from build123d import *

# Parameters (mm, degrees)
ESQUISSE1_W             = 4
ESQUISSE1_H             = 2
BASE_EXTRUSION_DEPTH    = 2
BOSS_EXTRU_1_DEPTH      = 0.5
BOSS_EXTRU_2_DEPTH      = 0.5
ESQUISSE4_W             = 5.5
ESQUISSE4_H             = 3.5
ESQUISSE5_W             = 4
ESQUISSE5_H             = 2
CONG_1_R                = 0.5
ESQUISSE6_W             = 2.5
ESQUISSE6_H             = 1
ENL_V_MAT_EXTRU_1_DEPTH = 8.5


with BuildPart() as part:
    # Esquisse1 → Base-Extrusion (new body)
    with BuildSketch(Plane.XY):
        Rectangle(ESQUISSE1_W, ESQUISSE1_H)
    extrude(amount=BASE_EXTRUSION_DEPTH)

    # Esquisse2 → Boss.-Extru.1 (add)
    with BuildSketch(Plane(origin=(0, 0, 0), x_dir=(-1, 0, 0), z_dir=(0, 0, -1))):
        with BuildLine():
            Line((-3, 2.5), (3, 2.5))
            ThreePointArc((3, 2.5), (3.353553391, 2.353553391), (3.5, 2))
            Line((3.5, 2), (3.5, -2))
            ThreePointArc((3.5, -2), (3.353553391, -2.353553391), (3, -2.5))
            Line((3, -2.5), (-3, -2.5))
            ThreePointArc((-3, -2.5), (-3.353553391, -2.353553391), (-3.5, -2))
            Line((-3.5, -2), (-3.5, 2))
            ThreePointArc((-3.5, 2), (-3.353553391, 2.353553391), (-3, 2.5))
        make_face()
    extrude(amount=BOSS_EXTRU_1_DEPTH)

    # Esquisse3 → Boss.-Extru.2 (add)
    with BuildSketch(Plane.XY.offset(2)):
        with BuildLine():
            Line((-3, -2.5), (3, -2.5))
            ThreePointArc((3, -2.5), (3.353553391, -2.353553391), (3.5, -2))
            Line((3.5, -2), (3.5, 2))
            ThreePointArc((3.5, 2), (3.353553391, 2.353553391), (3, 2.5))
            Line((3, 2.5), (-3, 2.5))
            ThreePointArc((-3, 2.5), (-3.353553391, 2.353553391), (-3.5, 2))
            Line((-3.5, 2), (-3.5, -2))
            ThreePointArc((-3.5, -2), (-3.353553391, -2.353553391), (-3, -2.5))
        make_face()
    extrude(amount=BOSS_EXTRU_2_DEPTH)

    # Esquisse4 → Boss.-Lissage1 section 0
    with BuildSketch(Plane.XY.offset(2.5)):
        Rectangle(ESQUISSE4_W, ESQUISSE4_H)
    # Esquisse5 → Boss.-Lissage1 section 1
    with BuildSketch(Plane.XY.offset(7)):
        Rectangle(ESQUISSE5_W, ESQUISSE5_H)
    loft()

    # Congé1
    cong_1_edges = [part.edges().sort_by_distance(p)[0] for p in [
        (-2.375, 1.375, 4.75),
        (2.375, 1.375, 4.75),
        (-2.375, -1.375, 4.75),
        (2.375, -1.375, 4.75),
    ]]
    fillet(cong_1_edges, radius=CONG_1_R)

    # Esquisse6 → Enlèv. mat.-Extru.1 (cut, through all)
    with BuildSketch(Plane.XY.offset(7)):
        Rectangle(ESQUISSE6_W, ESQUISSE6_H)
    extrude(amount=-ENL_V_MAT_EXTRU_1_DEPTH, mode=Mode.SUBTRACT)


solid = part.part
The model under review builds one solid part; all positions refer to its coordinate system, in mm. A direction names the side the tool comes from. Round coordinates to 2 decimals unless told otherwise and drop trailing zeros. Loops run counter-clockwise (first coordinate to the right, second up) from the corner with the lowest first, then second, coordinate; pieces in that order, holes last. Notation, with made-up numbers: (1, 55.25) -> (15, 55.25) arc R33 cw to (15, 84.25) -> close; hole circle Ø8 at (-16.5, 41). An arc over 180 degrees is marked (long way). One line per question, with ' | ' between items. Start each with the question number.
Item 1: Wall thickness on line 1 along Z through (x, y) = (3, -0.2); line 2 along Y through (x, z) = (0.75, 1); line 3 along X through (y, z) = (-0.1, 0.25): over which ranges is each line inside the solid? List them lowest first. Write a range as [from, to].
Item 2: For pin 1 (0.6 mm diameter, centred on x = 0, z = 0.5, fed in from +Y); pin 2 (1 mm diameter, centred on y = 0, z = 1, fed in from +X); pin 3 (3 mm diameter, centred on y = 1, z = 4.5, fed in from +X), all flat-tipped, find the tip position at first contact; note any pin that passes through.
Item 3: Add section A-A, the plane z = 1. Write out the cut boundary in (x, y).
Item 4: Machinability: for faces 1 (the face through (0, -2, 2.5)), 2 (the face through (-2, 0, 1)), 3 (the face through (0, 0.5, 3)), 4 (the face through (2, 0, 1)), which of the approach directions +Z, -Z, +X, -X, +Y, -Y give a long, thin tool a straight path to every point of the face, cutting with its end or side? Answer none if there is none.
Item 5: Draft analysis for pull direction Z (two halves, no side actions). For faces 5 (the face through (0, 1, -0.5)), 6 (the face through (-1.25, 0, 3)), 7 (the face through (0, 1, 1)), 8 (the face through (-0.4, 0.7, 7)), state which applies: +Z half, -Z half, draft (parallel to the pull), parting line (faces both ways), or undercut.
Return value:
1) line 1: z = [-0.5, 0], [2, 2.5] | line 2: y = [-1, -0.5], [0.5, 1] | line 3: x = [-2, -1.25], [1.25, 2]
2) pin 1: stops at y = 1 | pin 2: stops at x = 2 | pin 3: stops at x = 2.67
3) outline: (-2, -1) -> (2, -1) -> (2, 1) -> (-2, 1) -> close; hole (-1.25, -0.5) -> (1.25, -0.5) -> (1.25, 0.5) -> (-1.25, 0.5) -> close
4) face 1: +Z | face 2: -X, +Y, -Y | face 3: +Z, -Z | face 4: +X, +Y, -Y
5) face 5: -Z half | face 6: draft | face 7: undercut | face 8: +Z half
